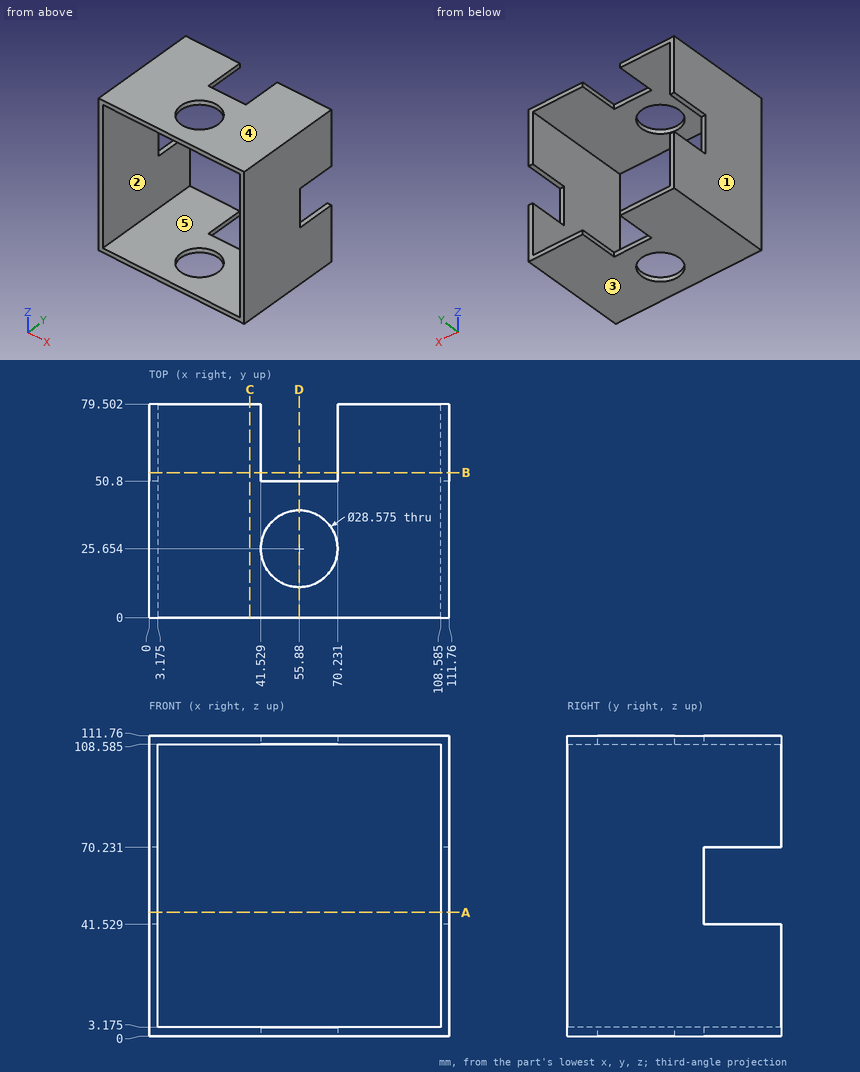
The figure shows three views and two pictorial views of one solid part (mm, origin at its lowest corner). Answer the questions. A direction names the side the tool comes from. Round coordinates to 2 decimals unless told otherwise and drop trailing zeros. Order: outer loops, then holes, each group sorted by start corner. A loop starts at its lowest first (then second) coordinate and runs counter-clockwise, first axis right, second up. Notation, with made-up numbers: M -9,66.5 L 13,66.5 A11 cw 13,70.5 Z; hole C -17.5,1 d7. An arc over 180 degrees is marked long. Answer in a Markdown table with one row per item. Add a question column.
1) Consider line 1 along Y through (x, z) = (55, 109); line 2 along Z through (x, y) = (91, 40) (3 decimals). Determine where each line is inside the solid, lowest interval first. Write a range as from..to.
2) A flat-ended cylindrical pin translates along its axis: pin 1 Ø3.5 at (x, z) = (50, 109.5) entering from +Y. Find the tip coordinate at first contact, or state that the pin passes through.
3) The part is cut by section C-C on x = 37.5. Determine the outline of the cut face in (y, z) (3 decimals), plus the area to 3 significant figures.
4) The part is cut by section D-D on x = 55.88. Determine the outline of the cut face in (y, z) (1 decimal), plus the area to 3 significant figures.
5) Which of the six approach directions +Z, -Z, +X, -X, +Y, -Y give full straight-line access (tool end or side, diameter ignored) to the marked faces 4 and 5?
6) The part is cut by section A-A on z = 46. Determine the outline of the cut face in (x, y) (3 decimals), plus the area to 3 significant figures.
7) The part is cut by section B-B on y = 54. Determine the outline of the cut face in (x, z) (3 decimals), plus the area to 3 significant figures.
8) Determine the mould class of the marked faces 1, 2 and 3 for opening direction X: pulls with the +X half, pulls with the -X half, needs draft (parallel to the pull), parting line crosses it, or undercut.
Findings below:
| question | item | result |
|---|---|---|
| 1 | line 1 | y = 0..11.39, 39.91..50.8 |
| 1 | line 2 | z = 0..3.175, 108.585..111.76 |
| 2 | pin 1 | stops at y = 50.8 |
| 3 | outline | M 0,0 L 79.502,0 L 79.502,3.175 L 0,3.175 Z; M 0,108.585 L 79.502,108.585 L 79.502,111.76 L 0,111.76 Z |
| 3 | area | 505 mm² |
| 4 | outline | M 0,0 L 11.4,0 L 11.4,3.2 L 0,3.2 Z; M 0,108.6 L 11.4,108.6 L 11.4,111.8 L 0,111.8 Z; M 39.9,0 L 50.8,0 L 50.8,3.2 L 39.9,3.2 Z; M 39.9,108.6 L 50.8,108.6 L 50.8,111.8 L 39.9,111.8 Z |
| 4 | area | 141 mm² |
| 5 | face 4 | +Z, +X, -X, +Y, -Y |
| 5 | face 5 | +Y, -Y |
| 6 | outline | M 0,0 L 3.175,0 L 3.175,50.8 L 0,50.8 Z; M 108.585,0 L 111.76,0 L 111.76,50.8 L 108.585,50.8 Z |
| 6 | area | 323 mm² |
| 7 | outline | M 0,0 L 41.529,0 L 41.529,3.175 L 3.175,3.175 L 3.175,41.529 L 0,41.529 Z; M 0,70.231 L 3.175,70.231 L 3.175,108.585 L 41.529,108.585 L 41.529,111.76 L 0,111.76 Z; M 70.231,0 L 111.76,0 L 111.76,41.529 L 108.585,41.529 L 108.585,3.175 L 70.231,3.175 Z; M 70.231,108.585 L 108.585,108.585 L 108.585,70.231 L 111.76,70.231 L 111.76,111.76 L 70.231,111.76 Z |
| 7 | area | 1,010 mm² |
| 8 | face 1 | pulls with the -X half |
| 8 | face 2 | undercut |
| 8 | face 3 | needs draft |
